from build123d import *
from OCP.BRepFilletAPI import BRepFilletAPI_MakeChamfer

# Parameters (mm, degrees)
SKETCH1_R           = 17.5
BOSS_EXTRUDE1_DEPTH = 46.433616
SKETCH2_R           = 13.379062462
CUT_EXTRUDE1_DEPTH  = 53.617304139
CHAMFER1_SIZE       = 0.480923
CHAMFER1_SIZE2      = 0.277661


with BuildPart() as part:
    # Sketch1 → Boss-Extrude1 (new body)
    with BuildSketch(Plane(origin=(0, 0, 0), x_dir=(1, 0, 0), z_dir=(0, 1, 0))):
        with Locations(Location((0, 0, 0), (0, 0, 270))):
            Circle(SKETCH1_R)
    extrude(amount=BOSS_EXTRUDE1_DEPTH)

    # Sketch2 → Cut-Extrude1 (cut, through all)
    with BuildSketch(Plane(origin=(0, 0, 0), x_dir=(1, 0, 0), z_dir=(0, 1, 0))):
        with Locations(Location((0, 0, 0), (0, 0, 270))):
            Circle(SKETCH2_R)
    extrude(amount=CUT_EXTRUDE1_DEPTH, mode=Mode.SUBTRACT)

    # Chamfer1: one chamfer whose edges measure the first distance from different faces: ONE call of the kernel's chamfer builder (chamfer() names one face for all edges)
    chamfer1_edges_1 = [part.edges().sort_by_distance(p)[0] for p in [
        (0, 0, -17.5),
    ]]
    chamfer1_side_1 = [part.faces().sort_by_distance(p)[0] for p in [
        (0, 0, -17.005025253),
    ]]
    chamfer1_edges_2 = [part.edges().sort_by_distance(p)[0] for p in [
        (0, 46.433616, -17.5),
    ]]
    chamfer1_side_2 = [part.faces().sort_by_distance(p)[0] for p in [
        (0, 23.216808, -17.5),
    ]]
    chamfer1_edges_3 = [part.edges().sort_by_distance(p)[0] for p in [
        (0, 0, -13.379062462),
    ]]
    chamfer1_side_3 = [part.faces().sort_by_distance(p)[0] for p in [
        (0, 23.216808, -13.379062462),
    ]]
    chamfer1_edges_4 = [part.edges().sort_by_distance(p)[0] for p in [
        (0, 46.433616, -13.379062462),
    ]]
    chamfer1_side_4 = [part.faces().sort_by_distance(p)[0] for p in [
        (0, 46.433616, -17.005025253),
    ]]
    chamfer1 = BRepFilletAPI_MakeChamfer(part.part.solid().wrapped)
    for e in chamfer1_edges_1:
        chamfer1.Add(CHAMFER1_SIZE, CHAMFER1_SIZE2, e.wrapped, chamfer1_side_1[0].wrapped)  # the first distance lies on this face
    for e in chamfer1_edges_2:
        chamfer1.Add(CHAMFER1_SIZE, CHAMFER1_SIZE2, e.wrapped, chamfer1_side_2[0].wrapped)  # the first distance lies on this face
    for e in chamfer1_edges_3:
        chamfer1.Add(CHAMFER1_SIZE, CHAMFER1_SIZE2, e.wrapped, chamfer1_side_3[0].wrapped)  # the first distance lies on this face
    for e in chamfer1_edges_4:
        chamfer1.Add(CHAMFER1_SIZE, CHAMFER1_SIZE2, e.wrapped, chamfer1_side_4[0].wrapped)  # the first distance lies on this face
    add(Compound.cast(chamfer1.Shape()), mode=Mode.REPLACE)


solid = part.part
Can you work these out from the model? Positions are in its coordinate system, mm. Round coordinates to 2 decimals unless told otherwise and drop trailing zeros. Write each loop counter-clockwise with the first axis right and the second up, starting at its lowest first coordinate (ties: lowest second). Pieces come first, ordered by that corner, then holes. Notation, with made-up numbers: (43, -20.5) -> (55, -20.5) arc R20 cw to (55, -16.5) -> close; hole circle Ø8 at (16, -25). An arc over 180 degrees is marked (long way). Use one line per item in the form item = value. Start each with the question number.
Q1. Imagine slicing it at B-B (x = 0). Please give me the cut outline in (y, z), then the cut area to 3 significant figures.
Q2. Imagine slicing it at C-C (y = 9.5). Please give me the cut outline in (x, z), then the cut area to 3 significant figures.
Q3. We'd pull the mould along X, two halves only. Please class faces 1 (the face through (-10.648, 22.795, -13.887)), 2 (the face through (8, 46.434, -12)), 3 (the face through (-13.06, 23, -2.9)): +X half, -X half, draft (parallel to the pull), parting line (faces both ways), or undercut.
Q4. Imagine slicing it at A-A (z = 0). Please give me the cut outline in (x, y).
Q5. I'm going to push flat-ended pins straight in: P1, Ø1.5, axis at x = 2, y = 29.5, coming from the +Z side; P2, Ø1.5, axis at y = 12.5, z = -2, coming from the -X side; P3, Ø1.5, axis at y = 39.5, z = -1.5, coming from the +X side. Where does each tip first touch, or does it pass through?
Q6. If I drill on probe 1 along X at (y, z) = (28, 0); probe 2 along Z at (x, y) = (-2, 28), over which ranges is the centre line in solid material (lowest first)? Write a range as [from, to].
Worked out:
q1.outline = (0, -17.02) -> (0.28, -17.5) -> (45.95, -17.5) -> (46.43, -17.22) -> (46.43, -13.86) -> (46.16, -13.38) -> (0.48, -13.38) -> (0, -13.66) -> close; (0, 13.66) -> (0.48, 13.38) -> (46.16, 13.38) -> (46.43, 13.86) -> (46.43, 17.22) -> (45.95, 17.5) -> (0.28, 17.5) -> (0, 17.02) -> close
q1.area = 382 mm^2
q2.outline = circle Ø35 at (0, 0); hole circle Ø26.76 at (0, 0)
q2.area = 400 mm^2
q3.face_1 = parting line
q3.face_2 = draft
q3.face_3 = undercut
q4.outline = (-17.5, 0.28) -> (-17.02, 0) -> (-13.66, 0) -> (-13.38, 0.48) -> (-13.38, 46.16) -> (-13.86, 46.43) -> (-17.22, 46.43) -> (-17.5, 45.95) -> close; (13.38, 0.48) -> (13.66, 0) -> (17.02, 0) -> (17.5, 0.28) -> (17.5, 45.95) -> (17.22, 46.43) -> (13.86, 46.43) -> (13.38, 46.16) -> close
q5.P1 = 17.46
q5.P2 = -17.46
q5.P3 = 17.48
q6.probe_1 = [-17.5, -13.38], [13.38, 17.5]
q6.probe_2 = [-17.39, -13.23], [13.23, 17.39]
